from build123d import *

# Parameters (mm, degrees)
SKETCH1_R           = 28.5
BOSS_EXTRUDE2_DEPTH = 8
SKETCH3_R           = 2.75
SKETCH3_R_2         = 1.6
BOSS_EXTRUDE3_DEPTH = 4.8
CUT_EXTRUDE1_START  = -8
SKETCH4_R           = 1.6
CUT_EXTRUDE1_DEPTH  = 8
SKETCH5_W           = 5
SKETCH5_H           = 72
BOSS_EXTRUDE4_DEPTH = 65
CIRPATTERN1_COUNT   = 4
SKETCH7_W           = 84.689019003
SKETCH7_H           = 34
CUT_EXTRUDE2_DEPTH  = 8
FILLET2_R           = 3
FILLET3_R           = 2
FILLET4_R           = 8


with BuildPart() as part:
    # Sketch1 → Boss-Extrude2 (new body)
    with BuildSketch(Plane(origin=(0, 0, 0), x_dir=(1, 0, 0), z_dir=(0, 1, 0))):
        with BuildLine():
            Line((0, 36), (50, 36))
            Line((50, 36), (50, -36))
            Line((50, -36), (0, -36))
            ThreePointArc((0, -36), (-36, 0), (0, 36))
        make_face()
        with Locations(Location((0, 0, 0), (0, 0, 270))):
            Circle(SKETCH1_R, mode=Mode.SUBTRACT)
        with BuildLine():
            Line((21.994317448, 28.5), (45, 28.5))
            Line((45, 28.5), (45, -28.5))
            Line((45, -28.5), (21.994317448, -28.5))
            ThreePointArc((21.994317448, -28.5), (36, 0), (21.994317448, 28.5))
        make_face(mode=Mode.SUBTRACT)
    extrude(amount=BOSS_EXTRUDE2_DEPTH)

    # Sketch3 → Boss-Extrude3 (add)
    with BuildSketch(Plane(origin=(0, 8, 0), x_dir=(1, 0, 0), z_dir=(0, 1, 0))):
        with Locations(Location((-22.273863607, 22.273863607, 0), (0, 0, 270))):
            Circle(SKETCH3_R)
        with Locations(Location((-22.273863607, 22.273863607, 0), (0, 0, 270))):
            Circle(SKETCH3_R_2, mode=Mode.SUBTRACT)
    boss_extrude3 = extrude(amount=BOSS_EXTRUDE3_DEPTH)

    # Sketch4 → Cut-Extrude1 (cut)
    with BuildSketch(Plane(origin=(0, 8, 0), x_dir=(1, 0, 0), z_dir=(0, 1, 0)).offset(CUT_EXTRUDE1_START)):
        with Locations(Location((-22.273863607, 22.273863607, 0), (0, 0, 270))):
            Circle(SKETCH4_R)
    cut_extrude1 = extrude(amount=CUT_EXTRUDE1_DEPTH, mode=Mode.SUBTRACT)

    # Sketch5 → Boss-Extrude4 (add)
    with BuildSketch(Plane(origin=(0, 8, 0), x_dir=(1, 0, 0), z_dir=(0, 1, 0))):
        with Locations((47.5, 0)):
            Rectangle(SKETCH5_W, SKETCH5_H)
    extrude(amount=BOSS_EXTRUDE4_DEPTH)

    # CirPattern1: Boss-Extrude3, Cut-Extrude1 ×4 about axis
    cirpattern1_axis = Axis((0, 0, 0), (0, 1, 0))
    add([boss_extrude3.rotate(cirpattern1_axis, i * 360 / CIRPATTERN1_COUNT) for i in range(1, CIRPATTERN1_COUNT)])
    add([cut_extrude1.rotate(cirpattern1_axis, i * 360 / CIRPATTERN1_COUNT) for i in range(1, CIRPATTERN1_COUNT)], mode=Mode.SUBTRACT)

    # Sketch7 → Cut-Extrude2 (cut)
    with BuildSketch(Plane.XZ):
        with Locations((-4.710445778, 0)):
            Rectangle(SKETCH7_W, SKETCH7_H)
    extrude(amount=-CUT_EXTRUDE2_DEPTH, mode=Mode.SUBTRACT)

    # Fillet2
    fillet2_edges = [part.edges().sort_by_distance(p)[0] for p in [
        (22.874658467, 4, -17),
        (-31.733263305, 4, -17),
        (31.733263305, 4, -17),
        (-31.733263305, 4, 17),
        (31.733263305, 4, 17),
        (22.874658467, 4, 17),
        (-22.874658467, 4, 17),
        (-22.874658467, 4, -17),
    ]]
    fillet(fillet2_edges, radius=FILLET2_R)

    # Fillet3
    fillet3_edges = [part.edges().sort_by_distance(p)[0] for p in [
        (21.994317448, 4, -28.5),
        (21.994317448, 4, 28.5),
    ]]
    fillet(fillet3_edges, radius=FILLET3_R)

    # Fillet4
    fillet4_edges = [part.edges().sort_by_distance(p)[0] for p in [
        (45, 8, -32.25),
        (45, 8, 32.25),
    ]]
    fillet(fillet4_edges, radius=FILLET4_R)


solid = part.part
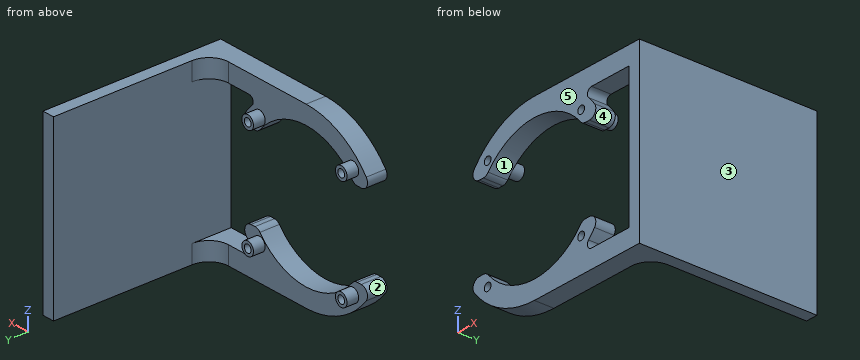
Check sheet for the modelled part. Datum: model origin and axes. Units: mm. Face numbers are marked on the shaded views. A direction names the side the tool comes from. Give positions to 0.01 mm unless a question says otherwise; leave off trailing zeros. Loops run counter-clockwise (first coordinate to the right, second up) from the corner with the lowest first, then second, coordinate; pieces in that order, holes last. Notation, with made-up numbers: M 63.5,-29 L 118.5,-29 A21 ccw 118.5,-14 Z; hole C 42,29.25 d4. An arc over 180 degrees is marked long. Answer as a JSON object with one key per item and string values. Group by question number.
Q1. Cross-section at D-D on x = 33.5. Record the cut outline in (y, z), then the cut area to 3 significant figures.
Q2. Release check for a two-part mould opening along X. For the marked faces 1, 2 and 3 record: released by +X, released by -X, zero draft, split by the parting line, or undercut.
Q3. Cross-section at A-A on x = 10.5. Record the cut outline in (y, z), then the cut area to 3 significant figures.
Q4. Cross-section at B-B on y = 24. Record the cut outline in (x, z).
Q5. Access from +Z, -Z, +X, -X, +Y, -Y to the whole of each face (thin tool, end or side, straight path). Record for the marked faces 4 and 5.
Q6. Material ranges on line 1 along X through (y, z) = (21.5, 32.5); line 2 along Y through (x, z) = (20, -21); line 3 along Y through (x, z) = (21, -31.5), recorded low to high. Write a range as [from, to].
Q7. Go/stop test with flat-tipped pins: P1, Ø2.5, axis at x = 22.27, z = -22.27, coming from the +Y side; P2, Ø1.6, axis at x = -21.5, z = -21.5, coming from the +Y side; P3, Ø15, axis at x = -11.5, z = 24.5, coming from the +Y side; P4, Ø8, axis at y = 37, z = 1, coming from the -X side. Record where each tip stops, or that it passes through.
Q8. Cross-section at C-C on z = -11. Record the cut outline in (x, y).
Evaluation:
{
 "1": {"outline": "M 0,-36 L 8,-36 L 8,-28.5 L 0,-28.5 Z; M 0,28.5 L 8,28.5 L 8,36 L 0,36 Z", "area": "120 mm2"},
 "2": {"face 1": "undercut", "face 2": "released by -X", "face 3": "released by +X"},
 "3": {"outline": "M 0,-36 L 8,-36 L 8,-26.5 L 0,-26.5 Z; M 0,26.5 L 8,26.5 L 8,36 L 0,36 Z", "area": "152 mm2"},
 "4": {"outline": "M 45,-36 L 50,-36 L 50,36 L 45,36 Z"},
 "5": {"face 4": "+Y, -Y", "face 5": "+Z, -Z, +X, -X, -Y"},
 "6": {"line 1": "x = [45, 50]", "line 2": "y = [0, 12.8]", "line 3": "y = [0, 8]"},
 "7": {"P1": "passes through", "P2": "stops at y = 12.8", "P3": "stops at y = 8", "P4": "stops at x = 45"},
 "8": {"outline": "M 45,0 L 50,0 L 50,73 L 45,73 Z"}
}
